Design review of the part built by this model. Coordinates are the model's own, in mm. A direction names the side the tool comes from. Give positions to 0.01 mm unless a question says otherwise; leave off trailing zeros. Order: outer loops, then holes, each group sorted by start corner. A loop starts at its lowest first (then second) coordinate and runs counter-clockwise, first axis right, second up. Notation, with made-up numbers: (-3.75, 30) -> (9.25, 30) arc R15 ccw to (9.25, 57) -> close; hole circle Ø10 at (-11, 50). An arc over 180 degrees is marked (long way). One line per item, written item: value. Start each with the question number.
1) Consider section D-D (y = -19). State the section outline as (x, z) points, plus the area to 3 significant figures.
2) Consider section C-C (z = 8). State the section outline as (x, y) points, plus the area to 3 significant figures.
3) Tool access review of faces 1 (the face through (16.5, 28, 17.9)), 2 (the face through (28, -16.5, 17.9)), 3 (the face through (-22, -30, 4)), 4 (the face through (15.024, 9.049, 26.535)): name each direction out of +Z, -Z, +X, -X, +Y, -Y from which nothing blocks a thin tool from reaching the whole face with its end or side.
4) Consider section A-A (z = 15). State the section outline as (x, y) points, plus the area to 3 significant figures.
5) Consider section B-B (x = 3). State the section outline as (y, z) points, plus the area to 3 significant figures.
6) Wall thickness on line 1 along Y through (x, z) = (0, 27.8); line 2 along X through (y, z) = (-27, 8); line 3 along Z through (x, y) = (8, -36.5): over which ranges is each line inside the solid? List them lowest first. Write a range as from..to.
7) For pin 1 (12 mm diameter, centred on x = -8, y = 21, fed in from -Z); pin 2 (3 mm diameter, centred on x = 21.5, z = 5, fed in from -Y); pin 3 (12 mm diameter, centred on y = -25.5, z = 15.5, fed in from -X), all flat-tipped, find the tip position at first contact; note any pin that passes through.
8) The part is to be moulded in two halves that separate along X. For faces 5 (the face through (-0.3, -32.5, 17.9)), 6 (the face through (-18.43, -41.4, -1.85)), 7 (the face through (-17.953, -9.434, 26.535)), say which applies: released by +X, released by -X, zero draft, split by the parting line, or undercut.
from build123d import *

# Parameters (mm, degrees)
SKETCH_W           = 60
SKETCH_H           = 60
SKETCH_R           = 2.25
PAD_DEPTH          = 9
FILLET_R           = 5
PAD001_DEPTH       = 18
SKETCH002_R        = 22.5
PAD002_DEPTH       = 2
SKETCH003_R        = 1.5
POCKET_DEPTH       = 5
POLARPATTERN_COUNT = 6
SKETCH004_R        = 14
POCKET001_DEPTH    = 29.001
SKETCH005_W        = 38
SKETCH005_H        = 28
PAD003_DEPTH       = 13
SKETCH006_W        = 38
SKETCH006_H        = 12
PAD004_DEPTH       = 9
FILLET001_R        = 2


with BuildPart() as part:
    # Sketch → Pad (new body)
    with BuildSketch(Plane.XY):
        Rectangle(SKETCH_W, SKETCH_H)
        with Locations((-25, 25)):
            Circle(SKETCH_R, mode=Mode.SUBTRACT)
        with Locations((25, 25)):
            Circle(SKETCH_R, mode=Mode.SUBTRACT)
        with Locations((25, -25)):
            Circle(SKETCH_R, mode=Mode.SUBTRACT)
        with Locations((-25, -25)):
            Circle(SKETCH_R, mode=Mode.SUBTRACT)
    extrude(amount=PAD_DEPTH)

    # Fillet
    fillet_edges = [part.edges().sort_by_distance(p)[0] for p in [
        (30, 30, 4.5),
        (-30, 30, 4.5),
        (-30, -30, 4.5),
        (30, -30, 4.5),
    ]]
    fillet(fillet_edges, radius=FILLET_R)

    # Sketch001 (on DatumPlane) → Pad001 (join)
    with BuildSketch(Plane.XY.offset(9)):
        with BuildLine():
            ThreePointArc((-25.590061, 20.034939), (-28.049199, 16.416225), (-30, 12.5))
            Line((-30, 12.5), (-30, -12.5))
            ThreePointArc((-30, -12.5), (-28.049199, -16.416225), (-25.590061, -20.034939))
            ThreePointArc((-20.034939, -25.590061), (-21.464466, -21.464466), (-25.590061, -20.034939))
            ThreePointArc((-20.034939, -25.590061), (0, -32.5), (20.034939, -25.590061))
            ThreePointArc((25.590061, -20.034939), (21.464466, -21.464466), (20.034939, -25.590061))
            ThreePointArc((25.590061, -20.034939), (28.049199, -16.416225), (30, -12.5))
            Line((30, -12.5), (30, 12.5))
            ThreePointArc((30, 12.5), (28.049199, 16.416225), (25.590061, 20.034939))
            ThreePointArc((20.034939, 25.590061), (21.464466, 21.464466), (25.590061, 20.034939))
            ThreePointArc((20.034939, 25.590061), (16.416225, 28.049199), (12.5, 30))
            Line((12.5, 30), (-12.5, 30))
            ThreePointArc((-12.5, 30), (-16.416225, 28.049199), (-20.034939, 25.590061))
            ThreePointArc((-25.590061, 20.034939), (-21.464466, 21.464466), (-20.034939, 25.590061))
        make_face()
    extrude(amount=PAD001_DEPTH)

    # Sketch002 (on Face17 of Pad001) → Pad002 (join)
    with BuildSketch(Plane.XY.offset(27)):
        Circle(SKETCH002_R)
    extrude(amount=PAD002_DEPTH)

    # Sketch003 (on Face32 of Pad002) → Pocket (cut)
    with BuildSketch(Plane.XY.offset(29)):
        with Locations((0, 19)):
            Circle(SKETCH003_R)
    pocket = extrude(amount=-POCKET_DEPTH, mode=Mode.SUBTRACT)

    # PolarPattern: Pocket ×6 about axis
    polarpattern_axis = Axis((0, 0, 29), (0, 0, 1))
    for i in range(1, POLARPATTERN_COUNT):
        add(pocket.rotate(polarpattern_axis, i * 360 / POLARPATTERN_COUNT), mode=Mode.SUBTRACT)

    # Sketch004 (on Face32 of PolarPattern) → Pocket001 (cut, through all)
    with BuildSketch(Plane.XY.offset(29)):
        Circle(SKETCH004_R)
    extrude(amount=-POCKET001_DEPTH, mode=Mode.SUBTRACT)

    # Sketch005 (on Face1 of Pocket001) → Pad003 (join)
    with BuildSketch(Plane(origin=(0, 0, 0), x_dir=(1, 0, 0), z_dir=(0, 0, -1))):
        with Locations((0, 28)):
            Rectangle(SKETCH005_W, SKETCH005_H)
    extrude(amount=PAD003_DEPTH)

    # Sketch006 (on Face21 of Pad003) → Pad004 (join)
    with BuildSketch(Plane(origin=(0, 0, 9), x_dir=(1, 0, 0), z_dir=(0, 0, -1))):
        with Locations((0, 36)):
            Rectangle(SKETCH006_W, SKETCH006_H)
    extrude(amount=PAD004_DEPTH)

    # Fillet001
    fillet001_edges = [part.edges().sort_by_distance(p)[0] for p in [
        (-19, -14, -6.5),
        (-19, -42, -2),
        (19, -42, -2),
        (19, -14, -6.5),
    ]]
    fillet(fillet001_edges, radius=FILLET001_R)


solid = part.part
Checked values:
1. outline: (-30, 0) -> (-19, 0) -> (-19, -13) -> (19, -13) -> (19, 0) -> (30, 0) -> (30, 9) -> (26.37, 9) -> (26.37, 27) -> (12.05, 27) -> (12.05, 29) -> (1.5, 29) -> (1.5, 24) -> (-1.5, 24) -> (-1.5, 29) -> (-12.05, 29) -> (-12.05, 27) -> (-26.37, 27) -> (-26.37, 9) -> (-30, 9) -> close
1. area: 2,020 mm^2
2. outline: (-30, -25) arc R5 ccw to (-25, -30) -> (-19, -30) -> (-19, -40) arc R2 ccw to (-17, -42) -> (17, -42) arc R2 ccw to (19, -40) -> (19, -30) -> (25, -30) arc R5 ccw to (30, -25) -> (30, 25) arc R5 ccw to (25, 30) -> (-25, 30) arc R5 ccw to (-30, 25) -> close; hole circle Ø4.5 at (-25, -25); hole circle Ø4.5 at (-25, 25); hole circle Ø28 at (0, 0); hole circle Ø4.5 at (25, -25); hole circle Ø4.5 at (25, 25)
2. area: 3,350 mm^2
3. face 1: +Z, +X, +Y
3. face 2: +Z, +X, -Y
3. face 3: +Z, -Z, -X, -Y
3. face 4: +Z
4. outline: (-30, -12.5) arc R32.5 ccw to (-25.59, -20.03) arc R5 cw to (-20.03, -25.59) arc R32.5 ccw to (20.03, -25.59) arc R5 cw to (25.59, -20.03) arc R32.5 ccw to (30, -12.5) -> (30, 12.5) arc R32.5 ccw to (25.59, 20.03) arc R5 cw to (20.03, 25.59) arc R32.5 ccw to (12.5, 30) -> (-12.5, 30) arc R32.5 ccw to (-20.03, 25.59) arc R5 cw to (-25.59, 20.03) arc R32.5 ccw to (-30, 12.5) -> close; hole circle Ø28 at (0, 0)
4. area: 2,530 mm^2
5. outline: (-42, -13) -> (-14, -13) -> (-14, 0) -> (-13.67, 0) -> (-13.67, 29) -> (-22.3, 29) -> (-22.3, 27) -> (-32.36, 27) -> (-32.36, 9) -> (-42, 9) -> close; (13.67, 0) -> (30, 0) -> (30, 27) -> (22.3, 27) -> (22.3, 29) -> (13.67, 29) -> close
5. area: 1,430 mm^2
6. line 1: y = -22.5..-20.5, -17.5..-14, 14..17.5, 20.5..22.5
6. line 2: x = -29.58..-26.03, -23.97..23.97, 26.03..29.58
6. line 3: z = -13..9
7. pin 1: stops at z = 0
7. pin 2: stops at y = -30
7. pin 3: stops at x = -26
8. face 5: split by the parting line
8. face 6: released by -X
8. face 7: undercut
